Autodesk Inventor part; units mm, degrees
ref_plane "YZ Plane" through (0, 0, 0) normal (1, 0, 0) x (0, 1, 0)
ref_plane "XZ Plane" through (0, 0, 0) normal (0, 1, 0) x (-1, 0, 0)
ref_plane "XY Plane" through (0, 0, 0) normal (0, 0, 1) x (1, 0, 0)
sketch "Sketch1" plane through (0, 0, 0) normal (0, 1, 0) x (-1, 0, 0)
  line L0 (13.2677, 19.6408) -> (-12.1323, 19.6408)
  line L1 (-12.1323, 19.6408) -> (-12.1323, -18.4592)
  line L2 (-12.1323, -18.4592) -> (13.2677, -18.4592)
  line L3 (13.2677, -18.4592) -> (13.2677, 19.6408)
  point P0 (0, 0)
  dimension "d0" = 25.4
  dimension "d1" = 38.1
extrude "Extrusion1" add sketch "Sketch1" along normal blind 3.175
hole "Hole1" at (-9.6799, 3.175, 14.8783) direction (0, -1, 0) diameter 4.4958 depth 3.175
hole "Hole2" at (8.5446, 3.175, 14.8783) direction (0, -1, 0) diameter 4.4958 depth 3.175
hole "Hole3" at (-9.6799, 3.175, -13.6967) direction (0, -1, 0) diameter 4.4958 depth 3.175
hole "Hole4" at (8.5446, 3.175, -13.6967) direction (0, -1, 0) diameter 4.4958 depth 3.175
hole "Hole6" at (-0.5677, 3.175, 8.8458) direction (0, -1, 0) diameter 3.175 depth 3.175
hole "Hole5" at (-0.5677, 3.175, -7.6642) direction (0, -1, 0) diameter 3.175 depth 3.175
hole "Hole7" at (-0.5677, 3.175, 0.5908) direction (0, -1, 0) diameter 6.985 depth 3.175
hole "Hole8" at (-0.5677, 3.175, 16.4658) direction (0, -1, 0) diameter 3.175 depth 3.175 tip angle 118
hole "Hole9" at (-0.5677, 3.175, -15.2842) direction (0, -1, 0) diameter 3.175 depth 3.175 tip angle 118
properties part number "Shield_3" material "Stainless Steel"
Can you work these out from the model? Positions are in its coordinate system, mm. Round coordinates to 2 decimals unless told otherwise and drop trailing zeros. Loops run counter-clockwise (first coordinate to the right, second up) from the corner with the lowest first, then second, coordinate; pieces in that order, holes last. Notation, with made-up numbers: (-16.75, 19) -> (14.25, 19) arc R25 ccw to (14.25, 42) -> close; hole circle Ø2 at (-16, -27.75). An arc over 180 degrees is marked (long way). Answer in a Markdown table with one row per item.
Item 1: Suppose I cut it at B-B, the plane x = -3. List the corners of the cut face in (y, z) for me (3 decimals).
Answer block:
| item | result |
|---|---|
| outline | (0, -18.459) -> (3.175, -18.459) -> (3.175, -1.915) -> (0, -1.915) -> close; (0, 3.097) -> (3.175, 3.097) -> (3.175, 19.641) -> (0, 19.641) -> close |
Item 2: Suppose I cut it at A-A, the plane z = -12.5. List the corners of the cut face in (x, y) for me (3 decimals), plus the area to 3 significant figures.
Answer block:
| item | result |
|---|---|
| outline | (-13.268, 0) -> (-11.583, 0) -> (-11.583, 3.175) -> (-13.268, 3.175) -> close; (-7.777, 0) -> (6.642, 0) -> (6.642, 3.175) -> (-7.777, 3.175) -> close; (10.447, 0) -> (12.132, 0) -> (12.132, 3.175) -> (10.447, 3.175) -> close |
| area | 56.5 mm² |
Item 3: Suppose I cut it at C-C, the plane z = 15.5. List the corners of the cut face in (x, y) for me (3 decimals).
Answer block:
| item | result |
|---|---|
| outline | (-13.268, 0) -> (-11.84, 0) -> (-11.84, 3.175) -> (-13.268, 3.175) -> close; (-7.52, 0) -> (-1.828, 0) -> (-1.828, 3.175) -> (-7.52, 3.175) -> close; (0.692, 0) -> (6.384, 0) -> (6.384, 3.175) -> (0.692, 3.175) -> close; (10.705, 0) -> (12.132, 0) -> (12.132, 3.175) -> (10.705, 3.175) -> close |
Item 4: If I drill on probe 1 along Z at (x, y) = (-0.5, 1); probe 2 along X at (y, z) = (0.5, 15.5); probe 3 along Z at (x, y) = (8.25, 2.2), over which ranges is the centre line in solid material (lowest first)?
Answer block:
| item | result |
|---|---|
| probe 1 | -18.46 to -16.87, -13.7 to -9.25, -6.08 to -2.9, 4.08 to 7.26, 10.43 to 14.88, 18.05 to 19.64 |
| probe 2 | -13.27 to -11.84, -7.52 to -1.83, 0.69 to 6.38, 10.7 to 12.13 |
| probe 3 | -18.46 to -15.93, -11.47 to 12.65, 17.11 to 19.64 |
Item 5: Suppose I cut it at D-D, the plane x = 7.75. List the corners of the cut face in (y, z) for me (3 decimals), plus the area to 3 significant figures.
Answer block:
| item | result |
|---|---|
| outline | (0, -18.459) -> (3.175, -18.459) -> (3.175, -15.799) -> (0, -15.799) -> close; (0, -11.594) -> (3.175, -11.594) -> (3.175, 12.776) -> (0, 12.776) -> close; (0, 16.981) -> (3.175, 16.981) -> (3.175, 19.641) -> (0, 19.641) -> close |
| area | 94.3 mm² |
Item 6: We'd pull the mould along Z, two halves only. Please class faces 1 (the flat face through (-1, 2, 19.641)), 2 (the flat face through (-13.268, 2, 0)), 3 (the cylindrical face through (-0.64, 1.57, -9.25)): released by +Z, released by -Z, zero draft, split by the parting line, or undercut.
Answer block:
| item | result |
|---|---|
| face 1 | released by +Z |
| face 2 | zero draft |
| face 3 | undercut |
